```python
from build123d import *

# Parameters (mm, degrees)
SKETCH1_R           = 39.624
SKETCH1_R_2         = 38.1
BOSS_EXTRUDE1_DEPTH = 381
SKETCH2_W           = 4.7625
SKETCH2_H           = 254
CUT_EXTRUDE1_DEPTH  = 386.098848027
CIRPATTERN1_COUNT   = 3


with BuildPart() as part:
    # Sketch1 → Boss-Extrude1 (new body)
    with BuildSketch(Plane(origin=(0, 0, 0), x_dir=(1, 0, 0), z_dir=(0, 1, 0))):
        with Locations(Location((0, 0, 0), (0, 0, 270))):
            Circle(SKETCH1_R)
        with Locations(Location((0, 0, 0), (0, 0, 270))):
            Circle(SKETCH1_R_2, mode=Mode.SUBTRACT)
    extrude(amount=BOSS_EXTRUDE1_DEPTH)

    # Sketch2 → Cut-Extrude1 (cut, through all)
    with BuildSketch(Plane.XY):
        with Locations((0, 127)):
            Rectangle(SKETCH2_W, SKETCH2_H)
    cut_extrude1 = extrude(amount=-CUT_EXTRUDE1_DEPTH, mode=Mode.SUBTRACT)

    # CirPattern1: Cut-Extrude1 ×3 about axis
    cirpattern1_axis = Axis((0, 0, 0), (0, 1, 0))
    for i in range(1, CIRPATTERN1_COUNT):
        add(cut_extrude1.rotate(cirpattern1_axis, i * 360 / CIRPATTERN1_COUNT), mode=Mode.SUBTRACT)


solid = part.part
```
The listing builds one solid part. Answer for the finished solid, in the listing's coordinates (mm). Coordinates: 2 decimals unless noted, no trailing zeros. Order: outer loops, then holes, each group sorted by start corner. A loop starts at its lowest first (then second) coordinate and runs counter-clockwise, first axis right, second up. Notation, with made-up numbers: M -32.75,24 L 26.25,24 A13 cw 26.25,35 Z; hole C -34,-21 d3. An arc over 180 degrees is marked long. Answer as a JSON object with one key per item and string values. Group by question number.
1. Section B-B on y = 146.5 is taken. Write down the section's boundary in (x, z), then the cut area to 3 significant figures.
2. Straight lines are drawn through the part: line 1 (X direction, y = 225, z = 0); line 2 (Z direction, x = -0.5, y = 113.5). For each, find the intervals that lie inside material, in ascending order.
3. Section C-C on x = 18 is taken. Write down the section's boundary in (y, z).
4. Determine the mould class of faces 1 (the cylindrical face through (11.44, 187.83, 36.34)), 2 (the cylindrical face through (11.902, 187.833, 37.794)), 3 (the flat face through (21, 381, -32)) for opening direction Z: released by +Z, released by -Z, zero draft, split by the parting line, or undercut.
5. Flat-ended cylindrical pins translate along their axes: P1, Ø3, axis at x = -8, y = 315.5, coming from the -Z side; P2, Ø10, axis at y = 253, z = -3, coming from the +X side; P3, Ø0.8, axis at x = 0.5, z = -38.5, coming from the -Y side; P4, Ø4, axis at x = 24, z = -25.5, coming from the -Y side. Find the tip coordinate at first contact, or state that the pin passes through.
6. Section A-A on z = 0 is taken. Write down the section's boundary in (x, y).
Values follow:
{
 "1": {"outline": "M -35.44,17.71 A39.62 ccw -2.38,-39.55 L -2.38,-38.03 A38.1 cw -34.12,16.95 Z; M -33.06,21.84 L -31.74,21.07 A38.1 cw 31.74,21.07 L 33.06,21.84 A39.62 ccw Z; M 2.38,-39.55 A39.62 ccw 35.44,17.71 L 34.12,16.95 A38.1 cw 2.38,-38.03 Z", "area": "350 mm2"},
 "2": {"line 1": "-39.62 to -38.1, 38.1 to 39.62", "line 2": "38.1 to 39.62"},
 "3": {"outline": "M 0,-35.3 L 381,-35.3 L 381,-33.58 L 0,-33.58 Z; M 0,33.58 L 381,33.58 L 381,35.3 L 0,35.3 Z"},
 "4": {"face 1": "undercut", "face 2": "split by the parting line", "face 3": "zero draft"},
 "5": {"P1": "z = -39.09", "P2": "x = 39.62", "P3": "y = 254", "P4": "through"},
 "6": {"outline": "M -39.62,0 L -38.1,0 L -38.1,381 L -39.62,381 Z; M 38.1,0 L 39.62,0 L 39.62,381 L 38.1,381 Z"}
}
